The listing builds one solid part. Answer for the finished solid, in the listing's coordinates (mm). Face numbers are marked on the shaded views. A direction names the side the tool comes from. Coordinates: 2 decimals unless noted, no trailing zeros. Write each loop counter-clockwise with the first axis right and the second up, starting at its lowest first coordinate (ties: lowest second). Pieces come first, ordered by that corner, then holes.
(1) For a pull along Z with two mould halves and no side action, classify the marked faces 1, 2 and 3 as +Z half, -Z half, draft (parallel to the pull), parting line (faces both ways), or undercut.
(2) The part is cut by section D-D on z = 17. Determine the outline of the cut face in (x, y).
(3) Which of the six approach directions +Z, -Z, +X, -X, +Y, -Y give full straight-line access (tool end or side, diameter ignored) to the marked faces 4, 5 and 6?
(4) The part is cut by section A-A on z = 63.5. Determine the outline of the cut face in (x, y), plus the area to 3 significant figures.
(5) The part is cut by section B-B on x = 170.5. Determine the outline of the cut face in (y, z).
(6) The part is cut by section C-C on y = -27. Determine the outline of the cut face in (x, z), plus the area to 3 significant figures.
(7) Straight lines are drawn through the part: line 1 (Y direction, x = 174, z = 63); line 2 (X direction, y = 58, z = 85.5); line 3 (Y direction, x = 73, z = 80.5). For each, find the intervals that lie inside material, in ascending order.
(8) Given P1, Ø23, axis at x = 74, z = 17, coming from the +Y side; P2, Ø1, axis at y = -20.5, z = 29, coming from the -X side; P3, Ø3, axis at x = 165.5, z = 31.5, coming from the -Y side, each flat-ended and moving along its own axis, determine where each tip first touches the part or whether it passes through.
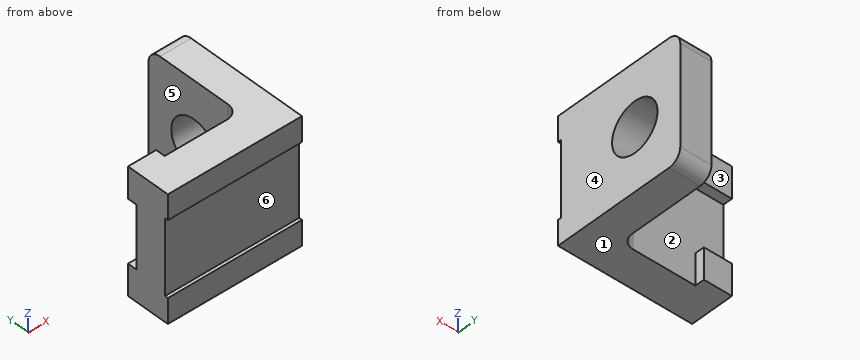
from build123d import *

# Parameters (mm, degrees)
BOSS_EXTRUDE1_DEPTH = 127
SKETCH2_R           = 25.4
CUT_EXTRUDE1_DEPTH  = 127
SKETCH3_W           = 76.2
SKETCH3_H           = 3.175
CUT_EXTRUDE2_DEPTH  = 199.564459386
SKETCH4_W           = 63.5
SKETCH4_H           = 9.525
CUT_EXTRUDE4_DEPTH  = 50.038
FILLET1_R           = 12.7


with BuildPart() as part:
    # Sketch1 → Boss-Extrude1 (new body)
    with BuildSketch(Plane.XY):
        Polygon((196.297790454, 68.2625), (196.297790454, -68.2625), (59.772790454, -68.2625), (59.772790454, -23.8125), (88.347790454, -23.8125), (88.347790454, -33.3375), (164.547790454, -33.3375), (164.547790454, 68.2625), align=None)
    extrude(amount=BOSS_EXTRUDE1_DEPTH)

    # Sketch2 → Cut-Extrude1 (cut)
    with BuildSketch(Plane(origin=(196.297790454, 0, 0), x_dir=(0, 0, -1), z_dir=(1, 0, 0))):
        with Locations(Location((-63.5, 17.4625, 0), (0, 0, 90))):
            Circle(SKETCH2_R)
    extrude(amount=-CUT_EXTRUDE1_DEPTH, mode=Mode.SUBTRACT)

    # Sketch3 → Cut-Extrude2 (cut, through all)
    with BuildSketch(Plane.ZY.offset(-59.772790454)):
        with Locations((63.5, -66.675)):
            Rectangle(SKETCH3_W, SKETCH3_H)
    extrude(amount=-CUT_EXTRUDE2_DEPTH, mode=Mode.SUBTRACT)

    # Sketch4 → Cut-Extrude4 (cut)
    with BuildSketch(Plane.ZY.offset(-59.772790454)):
        with Locations((63.5, -28.575)):
            Rectangle(SKETCH4_W, SKETCH4_H)
    extrude(amount=-CUT_EXTRUDE4_DEPTH, mode=Mode.SUBTRACT)

    # Fillet1
    fillet1_edges = [part.edges().sort_by_distance(p)[0] for p in [
        (180.422790454, 68.2625, 0),
        (164.547790454, -33.3375, 63.5),
        (180.422790454, 68.2625, 127),
    ]]
    fillet(fillet1_edges, radius=FILLET1_R)


solid = part.part
Model answer:
1. face 1: -Z half
1. face 2: undercut
1. face 3: draft
2. outline: (59.77, -68.26) - (196.3, -68.26) - (196.3, 68.26) - (164.55, 68.26) - (164.55, -20.64) arc R12.7 cw to (151.85, -33.34) - (88.35, -33.34) - (88.35, -23.81) - (59.77, -23.81) - close
3. face 4: +Z, -Z, +X, +Y, -Y
3. face 5: +Z, -Z, -X, +Y
3. face 6: +X, -X, -Y
4. outline: (59.77, -65.09) - (196.3, -65.09) - (196.3, -7.94) - (164.55, -7.94) - (164.55, -20.64) arc R12.7 cw to (151.85, -33.34) - (59.77, -33.34) - close; (164.55, 42.86) - (196.3, 42.86) - (196.3, 68.26) - (164.55, 68.26) - close
4. area: 5,980 mm2
5. outline: (-68.26, 0) - (55.56, 0) arc R12.7 ccw to (68.26, 12.7) - (68.26, 114.3) arc R12.7 ccw to (55.56, 127) - (-68.26, 127) - (-68.26, 101.6) - (-65.09, 101.6) - (-65.09, 25.4) - (-68.26, 25.4) - close; hole circle Ø50.8 at (17.46, 63.5)
6. outline: (59.77, 0) - (88.35, 0) - (88.35, 31.75) - (59.77, 31.75) - close; (59.77, 95.25) - (88.35, 95.25) - (88.35, 127) - (59.77, 127) - close; (162.84, 0) - (196.3, 0) - (196.3, 127) - (162.84, 127) - close
6. area: 6,060 mm2
7. line 1: y = -65.09 to -7.93, 42.86 to 68.26
7. line 2: x = 164.55 to 196.3
7. line 3: y = -65.09 to -33.34
8. P1: stops at y = -23.81
8. P2: stops at x = 164.54
8. P3: stops at y = -65.09
